Design review of the part built by this model. Coordinates are the model's own, in mm. A direction names the side the tool comes from. Coordinates: 2 decimals unless noted, no trailing zeros. Write each loop counter-clockwise with the first axis right and the second up, starting at its lowest first coordinate (ties: lowest second). Pieces come first, ordered by that corner, then holes.
Q1. Add section A-A, the plane z = -6.5. Give the boundary of the cut face in (x, y).
Q2. Add section C-C, the plane z = 8.5. Give the boundary of the cut face in (x, y) (3 decimals), plus the area to 3 significant figures.
Q3. To check wall thickness, follow probe 1 along Y at (x, z) = (1.3, 6); probe 2 along Z at (x, y) = (0.1, 4); probe 3 along Z at (x, y) = (0.3, -0.5). State the ranges of each line that lie inside material, in increasing order.
Q4. Add section D-D, the plane x = 0.6. Give the boundary of the cut face in (y, z) (3 decimals), plus the area to 3 significant figures.
Q5. The part is to be moulded in two halves that separate along Y. For faces 3 (the face through (1, -12, 9)), 4 (the face through (1, -2, 23)), 5 (the face through (1, -29.5, 2)), 6 (the face through (0.99, -3.4, -3.57)), say which applies: +Y half, -Y half, draft (parallel to the pull), parting line (faces both ways), or undercut.
Q6. Add section B-B, the plane y = -2.75. Give the boundary of the cut face in (x, z), plus the area to 3 significant figures.
Q7. Machinability: for faces 1 (the face through (1, -3, 3.5)), 2 (the face through (2, -2, 1)), which of the approach directions +Z, -Z, +X, -X, +Y, -Y give a long, thin tool a straight path to every point of the face, cutting with its end or side? Answer none if there is none.
Solid Edge part; units mm, degrees
sketch "Sketch1" plane through (0, 0, 0) normal (1, 0, 0) x (0, 1, 0)
  line L0 (25.5, -19.5) -> (25.5, 23)
  line L1 (25.5, 23) -> (-29.5, 23)
  line L2 (-29.5, 23) -> (-29.5, -19.5)
  line L3 (-29.5, -19.5) -> (25.5, -19.5)
extrude "Protrusion1" add sketch "Sketch1" along normal blind 2
sketch "Sketch2" plane through (0, 0, 0) normal (1, 0, 0) x (0, 1, 0)
  line L0 (6.5, 13.5) -> (-12, 13.5)
  line L1 (-12, 13.5) -> (-12, 3.5)
  line L2 (-12, 3.5) -> (6.5, 3.5)
  line L3 (6.5, 3.5) -> (6.5, 13.5)
  circle A0 centre (-15.245, 8.5) radius 1.98
  circle A1 centre (9.745, 8.5) radius 1.98
extrude "ExtrudedCutout_9" cut sketch "Sketch2" along normal blind 2
sketch "Sketch3" plane through (0, 0, 0) normal (1, 0, 0) x (0, 1, 0)
  circle A0 centre (-2.75, -6.5) radius 3
extrude "ExtrudedCutout_10" cut sketch "Sketch3" along normal blind 2
properties material "ABS Plastic, high impact"
Here are the results:
1. outline: (0, -29.5) - (2, -29.5) - (2, -5.75) - (0, -5.75) - close; (0, 0.25) - (2, 0.25) - (2, 25.5) - (0, 25.5) - close
2. outline: (0, -29.5) - (2, -29.5) - (2, -17.225) - (0, -17.225) - close; (0, -13.265) - (2, -13.265) - (2, -12) - (0, -12) - close; (0, 6.5) - (2, 6.5) - (2, 7.765) - (0, 7.765) - close; (0, 11.725) - (2, 11.725) - (2, 25.5) - (0, 25.5) - close
2. area: 57.2 mm2
3. probe 1: y = -29.5 to -12, 6.5 to 25.5
3. probe 2: z = -19.5 to 3.5, 13.5 to 23
3. probe 3: z = -19.5 to -8.48, -4.52 to 3.5, 13.5 to 23
4. outline: (-29.5, -19.5) - (25.5, -19.5) - (25.5, 23) - (-29.5, 23) - close; hole circle Ø3.96 at (-15.245, 8.5); hole (-12, 3.5) - (6.5, 3.5) - (6.5, 13.5) - (-12, 13.5) - close; hole circle Ø6 at (-2.75, -6.5); hole circle Ø3.96 at (9.745, 8.5)
4. area: 2,100 mm2
5. face 3: undercut
5. face 4: draft
5. face 5: -Y half
5. face 6: undercut
6. outline: (0, -19.5) - (2, -19.5) - (2, -9.5) - (0, -9.5) - close; (0, -3.5) - (2, -3.5) - (2, 3.5) - (0, 3.5) - close; (0, 13.5) - (2, 13.5) - (2, 23) - (0, 23) - close
6. area: 53.0 mm2
7. face 1: +X, -X
7. face 2: +Z, -Z, +X, +Y, -Y
